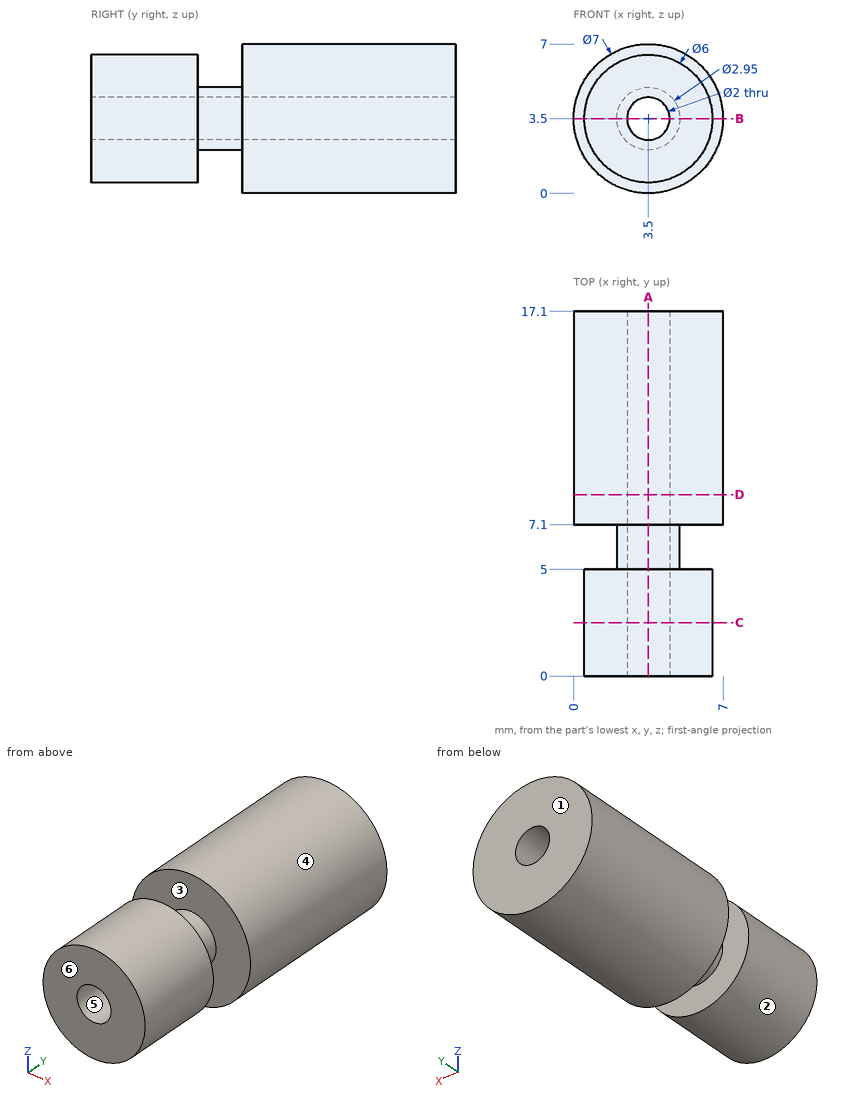
Answer from the drawing. Dimensions are ordinates in mm from the lowest x, y and z of the part. A direction names the side the tool comes from. Give positions to 0.01 mm unless a question says otherwise; leave off trailing zeros. Order: outer loops, then holes, each group sorted by start corner. A loop starts at its lowest first (then second) coordinate and runs counter-clockwise, first axis right, second up. Notation, with made-up numbers: (59, 78.5) -> (70, 78.5) arc R17 ccw to (70, 100.5) -> close; hole circle Ø5 at (46.5, 44.25). An arc over 180 degrees is marked (long way). Answer as a JSON object with one key per item and string values. Group by question number.
1. Section D-D on y = 8.5 is taken. Determine the outline of the cut face in (x, z).
2. Section B-B on z = 3.5 is taken. Determine the outline of the cut face in (x, y) (3 decimals), plus the area to 3 significant figures.
3. The mould has two halves that part along Z. Classify the marked faces 4, 5 and 6: released by +Z, released by -Z, zero draft, split by the parting line, or undercut.
4. Flat-ended cylindrical pins translate along their axes: pin 1 Ø2 at (y, z) = (15, 6) entering from -X; pin 2 Ø4 at (x, y) = (6, 5) entering from -Z; pin 3 Ø1.5 at (x, z) = (1, 4.5) entering from -Y; pin 4 Ø1.8 at (x, z) = (3.5, 3.5) entering from +Y. Find the tip coordinate at first contact, or state that the pin passes through.
5. A tool of negligible diameter and unlimited length cuts with its end or side. For the marked faces 1, 2 and 3, from which of +Z, -Z, +X, -X, +Y, -Y can it reach the whole face along a straight path? Write none if from no direction.
6. Consider line 1 along Z through (x, y) = (3.5, 13.75); line 2 along Y through (x, z) = (4.75, 5.75). Determine where each line is inside the solid, lowest interval first. Write a range as [from, to].
7. Section A-A on x = 3.5 is taken. Determine the outline of the cut face in (y, z) (3 decimals).
8. Section C-C on y = 2.5 is taken. Determine the outline of the cut face in (x, z), plus the area to 3 significant figures.
Result sheet:
{
 "1": {"outline": "circle Ø7 at (3.5, 3.5); hole circle Ø2 at (3.5, 3.5)"},
 "2": {"outline": "(0, 7.1) -> (2.025, 7.1) -> (2.025, 5) -> (0.5, 5) -> (0.5, 0) -> (2.5, 0) -> (2.5, 17.1) -> (0, 17.1) -> close; (4.5, 0) -> (6.5, 0) -> (6.5, 5) -> (4.975, 5) -> (4.975, 7.1) -> (7, 7.1) -> (7, 17.1) -> (4.5, 17.1) -> close", "area": "72.0 mm^2"},
 "3": {"face 4": "split by the parting line", "face 5": "undercut", "face 6": "zero draft"},
 "4": {"pin 1": "stops at x = 0.34", "pin 2": "stops at z = 0.54", "pin 3": "stops at y = 0", "pin 4": "passes through"},
 "5": {"face 1": "+Z, -Z, +X, -X, +Y", "face 2": "-Y", "face 3": "none"},
 "6": {"line 1": "z = [0, 2.5], [4.5, 7]", "line 2": "y = [0, 5], [7.1, 17.1]"},
 "7": {"outline": "(0, 0.5) -> (5, 0.5) -> (5, 2.025) -> (7.1, 2.025) -> (7.1, 0) -> (17.1, 0) -> (17.1, 2.5) -> (0, 2.5) -> close; (0, 4.5) -> (17.1, 4.5) -> (17.1, 7) -> (7.1, 7) -> (7.1, 4.975) -> (5, 4.975) -> (5, 6.5) -> (0, 6.5) -> close"},
 "8": {"outline": "circle Ø6 at (3.5, 3.5); hole circle Ø2 at (3.5, 3.5)", "area": "25.1 mm^2"}
}
